For this review, take the finished solid that the model builds, in its own axes (mm). Give positions to 0.01 mm unless a question says otherwise; leave off trailing zeros. Loops run counter-clockwise (first coordinate to the right, second up) from the corner with the lowest first, then second, coordinate; pieces in that order, holes last. Notation, with made-up numbers: (41.25, -30.5) - (91.25, -30.5) arc R14 cw to (91.25, -17.5) - close; hole circle Ø2 at (38.5, 68.5). An arc over 180 degrees is marked (long way). Use CSV: the item, a comma, the result in double quotes. Start each with the question number.
1. Wall thickness on line 1 (X direction, y = -1.5, z = 7); line 2 (Z direction, x = -27.5, y = -3.55); line 3 (Z direction, x = 27, y = -3.2): over which ranges is each line inside the solid? List them lowest first.
2. For pin 1 (1.5 mm diameter, centred on x = -4, y = -4.5, fed in from -Z); pin 2 (5.5 mm diameter, centred on x = -27.5, z = -29, fed in from -Y); pin 3 (3 mm diameter, centred on x = 27, z = 29, fed in from -Y), all flat-tipped, find the tip position at first contact; note any pin that passes through.
3. Take a section at A-A on z = -19. Give the boundary of the cut face in (x, y).
4. Take a section at D-D on x = -27.5. Give the boundary of the cut face in (y, z), plus the area to 3 significant figures.
5. Take a section at C-C on z = 1. Give the boundary of the cut face in (x, y).
6. Take a section at B-B on y = -3. Give the boundary of the cut face in (x, z).
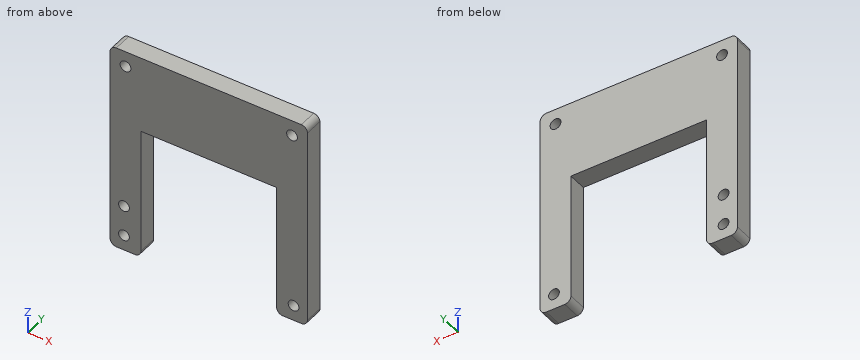
```python
from build123d import *

# Parameters (mm, degrees)
F0_W     = 64
F0_H     = 68
F1_DEPTH = 6
F2_R     = 1.75
F3_DEPTH = 25
F4_R     = 2


# Not quite as in the source:
# - a feature names something its author has since deleted; it is built from what else it names


with BuildPart() as f1:
    # F0 (on Front) → F1 (new body)
    with BuildSketch(Plane.XZ):
        Rectangle(F0_W, F0_H)
    extrude(amount=F1_DEPTH)

    # F2 (on face) → F3 (cut)
    with BuildSketch(Plane.XZ.offset(6)):
        Polygon((22, 9), (0, 9), (-22, 9), (-22, -34), (22, -34), align=None)
        with Locations((27.5, -29)):
            Circle(F2_R)
        with Locations((-27.5, -19)):
            Circle(F2_R)
        with Locations((-27.5, -29)):
            Circle(F2_R)
        with Locations((-27, 29)):
            Circle(F2_R)
        with Locations((27, 29)):
            Circle(F2_R)
    extrude(amount=-F3_DEPTH, mode=Mode.SUBTRACT)

    # F4
    f4_edges = [f1.edges().sort_by_distance(p)[0] for p in [
        (-32, -3, 34),
        (32, -3, 34),
        (-32, -3, -34),
        (32, -3, -34),
        (-22, -3, -34),
        (22, -3, -34),
    ]]
    fillet(f4_edges, radius=F4_R)


solid = f1.part
```
Check result:
1,line 1,"x = -32 to -22, 22 to 32"
1,line 2,"z = -34 to -30.75, -27.25 to -20.75, -17.25 to 27.32, 30.68 to 34"
1,line 3,"z = -34 to -30.68, -27.32 to 27.25, 30.75 to 34"
2,pin 1,"stops at z = 9"
2,pin 2,"stops at y = -6"
2,pin 3,"passes through"
3,outline,"(-32, -6) - (-29.25, -6) - (-29.25, 0) - (-32, 0) - close; (-25.75, -6) - (-22, -6) - (-22, 0) - (-25.75, 0) - close; (22, -6) - (32, -6) - (32, 0) - (22, 0) - close"
4,outline,"(-6, -34) - (0, -34) - (0, -30.75) - (-6, -30.75) - close; (-6, -27.25) - (0, -27.25) - (0, -20.75) - (-6, -20.75) - close; (-6, -17.25) - (0, -17.25) - (0, 27.32) - (-6, 27.32) - close; (-6, 30.68) - (0, 30.68) - (0, 34) - (-6, 34) - close"
4,area,"346 mm²"
5,outline,"(-32, -6) - (-22, -6) - (-22, 0) - (-32, 0) - close; (22, -6) - (32, -6) - (32, 0) - (22, 0) - close"
6,outline,"(-32, -32) arc R2 ccw to (-30, -34) - (-24, -34) arc R2 ccw to (-22, -32) - (-22, 9) - (22, 9) - (22, -32) arc R2 ccw to (24, -34) - (30, -34) arc R2 ccw to (32, -32) - (32, 32) arc R2 ccw to (30, 34) - (-30, 34) arc R2 ccw to (-32, 32) - close; hole circle Ø3.5 at (-27.5, -29); hole circle Ø3.5 at (-27.5, -19); hole circle Ø3.5 at (-27, 29); hole circle Ø3.5 at (27, 29); hole circle Ø3.5 at (27.5, -29)"
